Can you work these out from the drawing? Everything is in mm from the part's minimum corner. Coordinates: 2 decimals unless noted, no trailing zeros. Order: outer loops, then holes, each group sorted by start corner. A loop starts at its lowest first (then second) coordinate and runs counter-clockwise, first axis right, second up. Notation, with made-up numbers: (63, -29) - (121, -29) arc R29 ccw to (121, 8) - close; hole circle Ø11 at (56.25, 11). An arc over 180 degrees is marked (long way). Use a Markdown table: item, result. Add a question column.
(1) I want a section at A-A (z = 11). List the corners of the cut face in (x, y) for me, and give its area (3 significant figures).
(2) For pin 1 Ø11 at (x, z) = (376, 24) entering from +Y; pin 2 Ø15 at (y, z) = (264, 14.5) entering from +X, each with a flat end and sliding along its axis, tell me the tip position at first contact or that it passes through.
(3) If I drill on L1, parallel to Y at x = 160, z = 2; L2, parallel to Y at x = 94, z = 22; L3, parallel to X at y = 163, z = 20, over which ranges is the centre line in solid material (lowest first)? Write a range as [from, to].
(4) I want a section at C-C (y = 272). List the corners of the cut face in (x, z) for me.
(5) I want a section at B-B (x = 547). List the corners of the cut face in (y, z) for me.
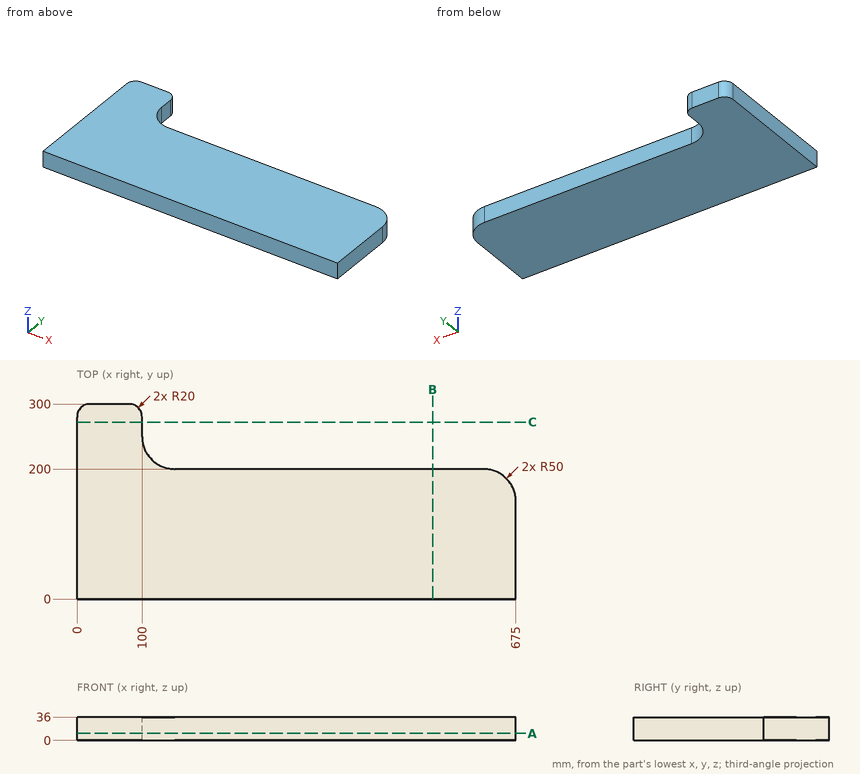
Answers follow:
| question | item | result |
|---|---|---|
| 1 | outline | (0, 0) - (675, 0) - (675, 150) arc R50 ccw to (625, 200) - (150, 200) arc R50 cw to (100, 250) - (100, 280) arc R20 ccw to (80, 300) - (20, 300) arc R20 ccw to (0, 280) - close |
| 1 | area | 145,000 mm² |
| 2 | pin 1 | stops at y = 200 |
| 2 | pin 2 | stops at x = 100 |
| 3 | L1 | y = [0, 200] |
| 3 | L2 | y = [0, 294.28] |
| 3 | L3 | x = [0, 673.28] |
| 4 | outline | (0, 0) - (100, 0) - (100, 36) - (0, 36) - close |
| 5 | outline | (0, 0) - (200, 0) - (200, 36) - (0, 36) - close |
